Work out the finished part from the listing and answer in its coordinate system (mm). Face numbers are marked on the shaded views. Give positions to 0.01 mm unless a question says otherwise; leave off trailing zeros. Order: outer loops, then holes, each group sorted by start corner. A loop starts at its lowest first (then second) coordinate and runs counter-clockwise, first axis right, second up. Notation, with made-up numbers: (-35, 51.5) - (-17, 51.5) arc R22 ccw to (-17, 70.5) - close; hole circle Ø8 at (45.25, -21.5). An arc over 180 degrees is marked (long way). Write each question's results on one line, items separated by ' | '.
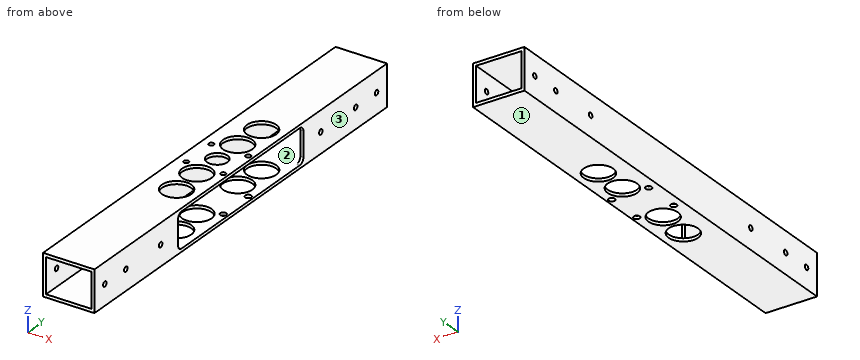
Autodesk Inventor part; units mm, degrees
ref_plane "YZ Plane" through (0, 0, 0) normal (1, 0, 0) x (0, 1, 0)
ref_plane "XZ Plane" through (0, 0, 0) normal (0, 1, 0) x (-1, 0, 0)
ref_plane "XY Plane" through (0, 0, 0) normal (0, 0, 1) x (1, 0, 0)
sketch "Sketch1" plane through (0, 0, 0) normal (0, 1, 0) x (-1, 0, 0)
  line L0 (0, 0) -> (50, 0)
  line L1 (50, 0) -> (50, -40)
  line L2 (50, -40) -> (0, -40)
  line L3 (0, -40) -> (0, 0)
  line L4 (3, -37) -> (47, -37)
  line L5 (47, -37) -> (47, -3)
  line L6 (47, -3) -> (3, -3)
  line L7 (3, -3) -> (3, -37)
  dimension "d0" = 50
  dimension "d1" = 40
  dimension "d2" = 3
extrude "Extrusion1" add sketch "Sketch1" along normal blind 420
sketch "Sketch2" plane through (0, 0, 0) normal (1, 0, 0) x (0, 0, -1)
  line L0 (0, 0) -> (40, 0)
  line L1 (40, 0) -> (40, 420)
  line L2 (0, 420) -> (40, 420)
  line L3 (0, 0) -> (0, 420)
  line L4 (3, 0) -> (3, 420)
  line L5 (37, 0) -> (37, 420)
  line L6 (3, 300) -> (37, 300)
  line L7 (37, 300) -> (37, 120)
  line L8 (37, 120) -> (3, 120)
  line L9 (3, 120) -> (3, 300)
  point P0 (3, 120)
  point P1 (37, 300)
  dimension "d5" = 120
  dimension "d6" = 120
extrude "Extrusion2" cut sketch "Sketch2" against normal blind 5 contours L4 L6 L5 L8
sketch "Sketch3" plane through (-50, 0, 0) normal (0, 0, 1) x (1, 0, 0)
  line L0 (0, 0) -> (50, 0)
  point P0 (27.2, 210)
  dimension "d9" = 210
  dimension "d10" = 27.2
hole "Hole1" at (-22.8, 210, 0) direction (0, 0, -1) diameter 19 depth 8 tip angle 118 counterbore diameter 20 counterbore depth 5
sketch "Sketch4" plane through (-50, 0, -3) normal (0, 0, 1) x (1, 0, 0)
  circle A0 centre (27.2, 210) radius 10
  circle A1 centre (27.2, 210) radius 25.4
  line L0 (8.6236, 227.3228) -> (44.5228, 228.5764)
  line L1 (44.5228, 228.5764) -> (45.7764, 192.6772)
  line L2 (45.7764, 192.6772) -> (9.8772, 191.4236)
  line L3 (9.8772, 191.4236) -> (8.6236, 227.3228)
  line L4 (8.6236, 227.3228) -> (45.7764, 192.6772) construction
  line L5 (44.5228, 228.5764) -> (9.8772, 191.4236) construction
  line L6 (50, 0) -> (50, 420)
  circle A2 centre (8.6236, 227.3228) radius 5.334
  circle A3 centre (44.5228, 228.5764) radius 5.334
  dimension "d18" = 50.8
  dimension "d19" = 2
  dimension "d34" = 10.668
  dimension "d35" = 10.668
hole "Hole2" [suppressed]
sketch "Sketch6" plane through (-3, 0, -3) normal (0, 0, -1) x (-1, 0, 0)
  circle A0 centre (37.1228, 191.4236) radius 5.334
  circle A1 centre (38.3764, 227.3228) radius 5.334
  circle A2 centre (2.4772, 228.5764) radius 5.334
  point P0 (-3, 0)
hole "Hole4" [suppressed]
sketch "Sketch7" plane through (0, 0, -40) normal (0, 0, -1) x (-1, 0, 0)
  circle A0 centre (22.8, 210) radius 10
  point P0 (0, 0)
  point P1 (22.8, 239.26)
  point P2 (22.8, 180.74)
  point P3 (21, 148.99)
  point P4 (21, 271.01)
  dimension "d45" = 31.75
  dimension "d46" = 1.8
  dimension "d47" = 31.75
  dimension "d94" = 29.26
  dimension "d95" = 29.26
hole "Hole5" at (-22.8, 239.26, -40) at (-22.8, 180.74, -40) at (-21, 148.99, -40) at (-21, 271.01, -40) direction (0, 0, 1) diameter 28.575 end through all
sketch "Sketch8" plane through (-3, 0, -3) normal (0, 0, -1) x (-1, 0, 0)
  circle A0 centre (19.8, 210) radius 25.4 construction
  line L0 (19.8, 210) -> (37.7605, 192.0395) construction
  line L1 (19.8, 210) -> (45.2, 210) construction
  circle A1 centre (19.8, 210) radius 10
  point P0 (-3, 0)
  point P1 (37.7605, 227.9605)
  point P2 (1.8395, 227.9605)
  point P3 (1.8395, 192.0395)
  dimension "d55" = 50.8
  dimension "d56" = 45
  dimension "d59" = 360
hole "Hole6" at (-40.7605, 192.0395, -3) at (-40.7605, 227.9605, -3) at (-4.8395, 227.9605, -3) at (-4.8395, 192.0395, -3) direction (0, 0, 1) diameter 5 end through all
sketch "Sketch9" plane through (0, 0, -40) normal (0, 0, -1) x (-1, 0, 0)
  circle A0 centre (40.7605, 227.9605) radius 2.5
  circle A1 centre (40.7605, 192.0395) radius 2.5
  circle A2 centre (4.8395, 227.9605) radius 2.5
  circle A3 centre (4.8395, 192.0395) radius 2.5
  point P0 (0, 0)
  point P1 (40.7605, 192.0395)
  point P2 (4.8395, 192.0395)
  point P3 (4.8395, 227.9605)
hole "Hole7" at (-40.7605, 227.9605, -40) at (-40.7605, 192.0395, -40) at (-4.8395, 192.0395, -40) at (-4.8395, 227.9605, -40) direction (0, 0, 1) diameter 6 depth 8 tip angle 118
fillet "Fillet1" radius 5 4 edges at (-1.5, 300, -37) (-1.5, 300, -3) (-1.5, 120, -37) (-1.5, 120, -3)
sketch "Sketch11" plane through (-50, 0, -40) normal (-1, 0, 0) x (0, 0, 1)
  circle A0 centre (20, 95) radius 2.5
  circle A1 centre (20, 375) radius 2.5
  circle A2 centre (20, 45) radius 2.5
  circle A3 centre (20, 15) radius 2.5
  circle A4 centre (20, 405) radius 2.5
  circle A5 centre (20, 325) radius 2.5
  arc A6 (-45, 37) -> (-40, 32) centre (-40, 37) ccw
  line L0 (-40, 32) -> (-25, 32)
  arc A7 (-20, 27) -> (-25, 32) centre (-25, 27) ccw
  line L1 (-20, 27) -> (-20, -3)
  line L2 (10, -3) -> (-20, -3)
  arc A8 (15, -8) -> (10, -3) centre (10, -8) ccw
  line L3 (15, -40) -> (15, -8)
  line L4 (145, -40) -> (15, -40)
  line L5 (145, 460) -> (145, -40)
  line L6 (15, 460) -> (145, 460)
  line L7 (15, 428) -> (15, 460)
  arc A9 (10, 423) -> (15, 428) centre (10, 428) ccw
  line L8 (-15, 423) -> (10, 423)
  arc A10 (-15, 423) -> (-20, 418) centre (-15, 418) ccw
  line L9 (-20, 418) -> (-20, 393)
  arc A11 (-25, 388) -> (-20, 393) centre (-25, 393) ccw
  line L10 (-25, 388) -> (-40, 388)
  arc A12 (-40, 388) -> (-45, 383) centre (-40, 383) ccw
  line L11 (-45, 383) -> (-45, 318)
  arc A13 (-50, 313) -> (-45, 318) centre (-50, 318) ccw
  line L12 (-50, 313) -> (-113, 313)
  arc A14 (-118, 318) -> (-113, 313) centre (-113, 318) ccw
  line L13 (-118, 318) -> (-118, 418)
  arc A15 (-118, 418) -> (-123, 423) centre (-123, 418) ccw
  line L14 (-630, 423) -> (-123, 423)
  arc A16 (-635, 428) -> (-630, 423) centre (-630, 428) ccw
  line L15 (-635, 460) -> (-635, 428)
  line L16 (-755, 460) -> (-635, 460)
  line L17 (-755, -40) -> (-755, 460)
  line L18 (-635, -40) -> (-755, -40)
  line L19 (-635, -8) -> (-635, -40)
  arc A17 (-630, -3) -> (-635, -8) centre (-630, -8) ccw
  line L20 (-118, -3) -> (-630, -3)
  line L21 (-118, -3) -> (-118, 102)
  arc A18 (-113, 107) -> (-118, 102) centre (-113, 102) ccw
  line L22 (-113, 107) -> (-50, 107)
  arc A19 (-45, 102) -> (-50, 107) centre (-50, 102) ccw
  line L23 (-45, 102) -> (-45, 37)
  circle A20 centre (68.5, 440) radius 3
  circle A21 centre (68.5, -20) radius 3
  circle A22 centre (-742.5, 410) radius 2.5
  circle A23 centre (-742.5, 210) radius 2.5
  circle A24 centre (-742.5, 10) radius 2.5
  circle A25 centre (132.5, 310) radius 2.5
  circle A26 centre (132.5, 110) radius 2.5
  circle A27 centre (-305, 12.5) radius 2.5
  circle A28 centre (-485, 12.5) radius 2.5
  circle A29 centre (-485, 407.5) radius 2.5
  circle A30 centre (-305, 407.5) radius 2.5
  circle A31 centre (-125, 407.5) radius 2.5
  circle A32 centre (-125, 12.5) radius 2.5
  circle A33 centre (132.5, 10) radius 2.5
  circle A34 centre (132.5, 210) radius 2.5
  circle A35 centre (132.5, 410) radius 2.5
  circle A36 centre (-742.5, 110) radius 2.5
  circle A37 centre (-742.5, 310) radius 2.5
  circle A38 centre (33.5, -20) radius 3
  circle A39 centre (33.5, 440) radius 3
  arc A40 (40, 115) -> (35, 120) centre (35, 115) ccw
  line L24 (8, 120) -> (35, 120)
  arc A41 (3, 125) -> (8, 120) centre (8, 125) ccw
  line L25 (3, 295) -> (3, 125)
  arc A42 (8, 300) -> (3, 295) centre (8, 295) ccw
  line L26 (35, 300) -> (8, 300)
  arc A43 (35, 300) -> (40, 305) centre (35, 305) ccw
  line L27 (40, 393.2461) -> (40, 305)
  arc A44 (41.0957, 396.3696) -> (40, 393.2461) centre (45, 393.2461) ccw
  line L28 (58.4988, 418.1235) -> (41.0957, 396.3696)
  arc A45 (62.4031, 420) -> (58.4988, 418.1235) centre (62.4031, 415) ccw
  line L29 (115, 420) -> (62.4031, 420)
  arc A46 (120, 415) -> (115, 420) centre (115, 415) ccw
  line L30 (120, 5) -> (120, 415)
  arc A47 (115, 0) -> (120, 5) centre (115, 5) ccw
  line L31 (62.4031, 0) -> (115, 0)
  arc A48 (58.4988, 1.8765) -> (62.4031, 0) centre (62.4031, 5) ccw
  line L32 (41.0957, 23.6304) -> (58.4988, 1.8765)
  arc A49 (40, 26.7539) -> (41.0957, 23.6304) centre (45, 26.7539) ccw
  line L33 (40, 115) -> (40, 26.7539)
  point P0 (40, 0)
  point P1 (20, 405)
  point P2 (20, 375)
  point P3 (20, 325)
  point P4 (20, 95)
  point P5 (20, 45)
  point P6 (20, 15)
hole "Hole8" at (-50, 405, -20) at (-50, 375, -20) at (-50, 325, -20) at (-50, 95, -20) at (-50, 45, -20) at (-50, 15, -20) direction (1, 0, 0) diameter 5 end through all
equation "\"d6\" = d5"
properties part number "Wasp Mount Bar"
1. A cutting plane is placed at C-C, the plane y = 148.99. Write down the section's boundary in (x, z), then the cut area to 3 significant figures.
Answer list:
outline: (-50, -40) - (-35.29, -40) - (-35.29, -37) - (-47, -37) - (-47, -3) - (-35.29, -3) - (-35.29, 0) - (-50, 0) - close; (-6.71, -40) - (0, -40) - (0, -37) - (-6.71, -37) - close; (-6.71, -3) - (0, -3) - (0, 0) - (-6.71, 0) - close | area: 231 mm^2
2. Determine the mould class of the marked faces 1, 2 and 3 for opening direction X: +X half, -X half, draft (parallel to the pull), parting line (faces both ways), or undercut.
Answer list:
face 1: draft | face 2: undercut | face 3: +X half
3. A cutting plane is placed at A-A, the plane z = -26. Write down the section's boundary in (x, y).
Answer list:
outline: (-50, 0) - (-47, 0) - (-47, 420) - (-50, 420) - close; (-3, 0) - (0, 0) - (0, 120) - (-3, 120) - close; (-3, 300) - (0, 300) - (0, 420) - (-3, 420) - close
4. A cutting plane is placed at B-B, the plane y = 210. Write down the section's boundary in (x, z).
Answer list:
outline: (-50, -40) - (0, -40) - (0, -37) - (-47, -37) - (-47, -3) - (-32.8, -3) - (-32.8, 0) - (-50, 0) - close; (-12.8, -3) - (0, -3) - (0, 0) - (-12.8, 0) - close
5. Straight lines are drawn through the part: line 1 (Z direction, x = -1, y = 15); line 2 (Z direction, x = -45.5, y = 20.5); line 3 (X direction, y = 307, z = -18). For each, find the intervals that lie inside material, in ascending order. Write a range as [from, to].
Answer list:
line 1: [-40, -22.5], [-17.5, 0] | line 2: [-40, -37], [-3, 0] | line 3: [-50, -47], [-3, 0]
